```python
from build123d import *

# Parameters (mm, degrees)
F0_R            = 15.5
F1_DEPTH        = 10
F2_R            = 4
F3_DEPTH        = 25
F3_COPIES_COUNT = 6


# Not quite as in the source:
# - a pattern or mirror of a feature is missing from the dataset's text; its kind, count and spacing are read off the source's solid


with BuildPart() as f1:
    # F0 (on Top) → F1 (new body)
    with BuildSketch(Plane.XY):
        with BuildLine():
            ThreePointArc((115, 0), (81.3172798365, 81.3172798365), (0, 115))
            ThreePointArc((0, 115), (-81.3172798365, -81.3172798365), (115, 0))
        make_face()
        with BuildLine():
            ThreePointArc((79.8738727668, -29.0717121827), (-29.6258097027, -79.6700156863), (-79.4623147975, 30.1784778779))
            Line((-79.4623147975, 30.1784778779), (-74.7757231643, 28.4357385213))
            ThreePointArc((-74.7757231643, 28.4357385213), (-28.4357385213, -74.7757231643), (74.7757231643, -28.4357385213))
            Line((74.7757231643, -28.4357385213), (79.8738727668, -29.0717121827))
        make_face(mode=Mode.SUBTRACT)
        with BuildLine():
            Line((-42.1306922898, 42.7200745222), (-38.6198012657, 39.160068312))
            ThreePointArc((-38.6198012657, 39.160068312), (-39.160068312, -38.6198012657), (38.6198012657, -39.160068312))
            Line((38.6198012657, -39.160068312), (42.1306922898, -42.7200745222))
            ThreePointArc((42.1306922898, -42.7200745222), (-42.7200745222, -42.1306922898), (-42.1306922898, 42.7200745222))
        make_face(mode=Mode.SUBTRACT)
        Circle(F0_R, mode=Mode.SUBTRACT)
        with BuildLine():
            ThreePointArc((-24.5762371691, 24.9200434713), (24.9200434713, 24.5762371691), (24.5762371691, -24.9200434713))
            Line((24.5762371691, -24.9200434713), (21.0653461449, -21.3600372611))
            ThreePointArc((21.0653461449, -21.3600372611), (21.3600372611, 21.0653461449), (-21.0653461449, 21.3600372611))
            Line((-21.0653461449, 21.3600372611), (-24.5762371691, 24.9200434713))
        make_face(mode=Mode.SUBTRACT)
    extrude(amount=F1_DEPTH)

    # F2 (on face) → F3 (cut)
    with BuildSketch(Plane.XY.offset(10)):
        with Locations((0, 105)):
            Circle(F2_R)
    f3 = extrude(amount=-F3_DEPTH, mode=Mode.SUBTRACT)

    # F3_copies: F3 ×6 about axis
    f3_copies_axis = Axis((0, 0, 0), (0, 0, 1))
    for i in range(1, F3_COPIES_COUNT):
        add(f3.rotate(f3_copies_axis, i * 360 / F3_COPIES_COUNT), mode=Mode.SUBTRACT)


solid = f1.part
```
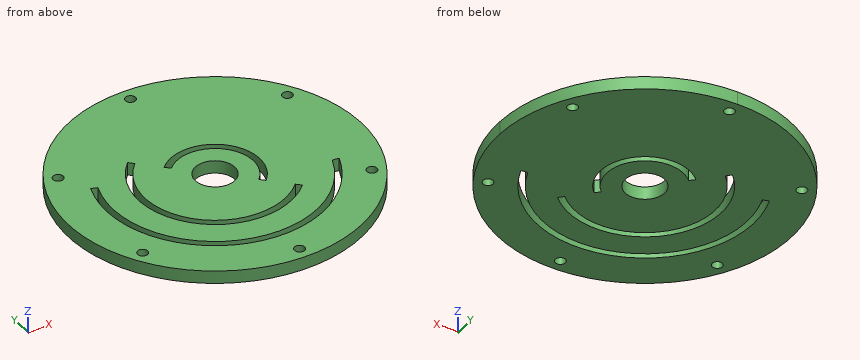
The model under review builds one solid part; all positions refer to its coordinate system, in mm. Give positions to 0.01 mm unless a question says otherwise; leave off trailing zeros. Loops run counter-clockwise (first coordinate to the right, second up) from the corner with the lowest first, then second, coordinate; pieces in that order, holes last. Notation, with made-up numbers: (40.25, 0) -> (48.25, 0) arc R31 ccw to (48.25, 35) -> close; hole circle Ø8 at (-4, 50). An arc over 180 degrees is marked (long way). Use CSV: the item, a comma, the result in double quotes.
1. For P1, Ø1.5, axis at x = -34, z = 8, coming from the +Y side; P2, Ø5, axis at y = -57.5, z = 3, coming from the -X side; P3, Ø2, axis at y = 71.5, z = 5, coming from the +X side, all flat-tipped, find the tip position at first contact; note any pin that passes through.
Result:
P1,"stops at y = 110.09"
P2,"stops at x = -101"
P3,"stops at x = 90.86"
2. Consider section D-D, the plane y = 52. Write out the cut boundary in (x, z), then the cut area to 3 significant figures.
Result:
outline,"(-102.57, 0) -> (-94.9, 0) -> (-94.9, 10) -> (-102.57, 10) -> close; (-86.96, 0) -> (86.96, 0) -> (86.96, 10) -> (-86.96, 10) -> close; (94.9, 0) -> (102.57, 0) -> (102.57, 10) -> (94.9, 10) -> close"
area,"1,890 mm²"
3. Consider section C-C, the plane y = -105. Write out the cut boundary in (x, z).
Result:
outline,"(-46.9, 0) -> (-4, 0) -> (-4, 10) -> (-46.9, 10) -> close; (4, 0) -> (46.9, 0) -> (46.9, 10) -> (4, 10) -> close"
4. Consider section B-B, the plane z = 7. Count the separate pieces of the cut face and the enclosed holes in it, then the cut area to 3 significant figures.
Result:
separate pieces,"1"
enclosed holes,"10"
area,"37,800 mm²"
5. To check wall thickness, follow probe 1 along X at (y, z) = (-23, 8.5); probe 2 along Y at (x, z) = (-21, 7.25); probe 3 along Y at (x, z) = (-47, 3.75). State the ranges of each line that lie inside material, in increasing order. Write a range as from..to.
Result:
probe 1,"x = -112.68..-81.83, -76.62..-55.42, -49.96..22.68, 26.38..112.68"
probe 2,"y = -113.07..-82.37, -77.19..-56.2, -50.83..21.42, 28..113.07"
probe 3,"y = -104.96..-70.82, -64.74..-37.3, -28.57..28.57, 37.3..104.96"
6. Consider section A-A, the plane y = -12. Write out the cut boundary in (x, z), then the cut area to 3 significant figures.
Result:
outline,"(-114.37, 0) -> (-84.15, 0) -> (-84.15, 10) -> (-114.37, 10) -> close; (-79.09, 0) -> (-58.79, 0) -> (-58.79, 10) -> (-79.09, 10) -> close; (-53.67, 0) -> (-9.81, 0) -> (-9.81, 10) -> (-53.67, 10) -> close; (9.81, 0) -> (27.5, 0) -> (27.5, 10) -> (9.81, 10) -> close; (32.88, 0) -> (114.37, 0) -> (114.37, 10) -> (32.88, 10) -> close"
area,"1,940 mm²"
